Here's how the part is built. I have some questions about the finished solid (model axes, mm). Face numbers are marked on the shaded views. A direction names the side the tool comes from. Coordinates: 2 decimals unless noted, no trailing zeros. Write each loop counter-clockwise with the first axis right and the second up, starting at its lowest first coordinate (ties: lowest second). Pieces come first, ordered by that corner, then holes.
Item 1: I'm going to push flat-ended pins straight in: pin 1 Ø10 at (x, y) = (-18, 30) entering from -Z; pin 2 Ø4 at (y, z) = (29.5, 4) entering from -X; pin 3 Ø5.5 at (x, z) = (58.67, 4.78) entering from +Y; pin 4 Ø4.5 at (x, z) = (19.56, 4.95) entering from -Y. Where does each tip first touch, or does it pass through?
Item 2: If I drill on line 1 (X direction, y = 49, z = 5); line 2 (X direction, y = 45.5, z = 4.5); line 3 (Y direction, x = 19.5, z = 2), over which ranges is the centre line in solid material (lowest first)?
Item 3: If we section it at D-D (y = 31): Please give me the cut outline in (x, z), then the cut area to 3 significant figures.
Item 4: For the marked faces 1, 2 and 3, which set-ups out of +Z, -Z, +X, -X, +Y, -Y let a thin tool reach every point of the face, with its end or its side?
Item 5: If we section it at B-B (x = -55.5): Please give me the cut outline in (y, z), then the cut area to 3 significant figures.
Item 6: If we section it at A-A (y = 25): Please give me the cut outline in (x, z), then the cut area to 3 significant figures.
Item 7: If we section it at C-C (y = 50.5): Please give me the cut outline in (x, z), then the cut area to 3 significant figures.
from build123d import *
from build123d import SkipClean  # not in build123d's __all__

# Parameters (mm, degrees)
F1_DEPTH       = 10
F3_D           = 3.556
F3_CBORE_D     = 7.62
F3_CBORE_DEPTH = 13.75
F4_DEPTH       = 10.0010001
F6_D           = 3.556
F7_R           = 5


with BuildPart() as f1:
    # F0 (on Top) → F1 (new body)
    with BuildSketch(Plane.XY):
        with BuildLine():
            ThreePointArc((30, 32.8671568591), (40.2999174323, 18.8723780946), (44.4550334608, 2))
            Line((44.4550334608, 2), (44.4550334608, 7))
            Line((44.4550334608, 7), (49.002550954, 7))
            ThreePointArc((49.002550954, 7), (42.6890737127, 25.0577929106), (30, 39.3732142452))
            Line((30, 39.3732142452), (30, 32.8671568591))
        make_face()
        with BuildLine():
            ThreePointArc((20.7364413533, 39.3732142452), (25.5759421328, 36.4159468368), (30, 32.8671568591))
            Line((30, 32.8671568591), (30, 39.3732142452))
            Line((30, 39.3732142452), (20.7364413533, 39.3732142452))
        make_face()
        with BuildLine():
            ThreePointArc((-20.7364413533, 39.3732142452), (0, 44.5), (20.7364413533, 39.3732142452))
            Line((20.7364413533, 39.3732142452), (30, 39.3732142452))
            ThreePointArc((30, 39.3732142452), (15.8315491079, 46.9000218853), (-1.83e-08, 49.5))
            ThreePointArc((-1.83e-08, 49.5), (-15.8315491253, 46.9000218795), (-30, 39.3732142452))
            Line((-30, 39.3732142452), (-20.7364413533, 39.3732142452))
        make_face()
        with BuildLine():
            Line((-30, 39.3732142452), (-30, 32.8671568591))
            ThreePointArc((-30, 32.8671568591), (-25.5759421328, 36.4159468368), (-20.7364413533, 39.3732142452))
            Line((-20.7364413533, 39.3732142452), (-30, 39.3732142452))
        make_face()
        with BuildLine():
            ThreePointArc((-44.4550334608, 2), (-40.2999174323, 18.8723780946), (-30, 32.8671568591))
            Line((-30, 32.8671568591), (-30, 39.3732142452))
            ThreePointArc((-30, 39.3732142452), (-42.6890737127, 25.0577929106), (-49.002550954, 7))
            Line((-49.002550954, 7), (-44.4550334608, 7))
            Line((-44.4550334608, 7), (-44.4550334608, 2))
        make_face()
        with BuildLine():
            Line((-64.4550334608, 2), (-49.4595794564, 2))
            ThreePointArc((-49.4595794564, 2), (-49.2945005172, 4.5057983491), (-49.002550954, 7))
            Line((-49.002550954, 7), (-64.4550334608, 7))
            Line((-64.4550334608, 7), (-64.4550334608, 2))
        make_face()
        with BuildLine():
            Line((-49.4595794564, 2), (-44.4550334608, 2))
            Line((-44.4550334608, 2), (-44.4550334608, 7))
            Line((-44.4550334608, 7), (-49.002550954, 7))
            ThreePointArc((-49.002550954, 7), (-49.2945005172, 4.5057983491), (-49.4595794564, 2))
        make_face()
        with BuildLine():
            Line((44.4550334608, 7), (44.4550334608, 2))
            Line((44.4550334608, 2), (49.4595794564, 2))
            ThreePointArc((49.4595794564, 2), (49.2945005172, 4.5057983491), (49.002550954, 7))
            Line((49.002550954, 7), (44.4550334608, 7))
        make_face()
        with BuildLine():
            ThreePointArc((49.002550954, 7), (49.2945005172, 4.5057983491), (49.4595794564, 2))
            Line((49.4595794564, 2), (64.4550334608, 2))
            Line((64.4550334608, 2), (64.4550334608, 7))
            Line((64.4550334608, 7), (49.002550954, 7))
        make_face()
        with BuildLine():
            Line((-30, 49.5), (-30, 39.3732142452))
            ThreePointArc((-30, 39.3732142452), (-15.8315491253, 46.9000218795), (-1.83e-08, 49.5))
            Line((-1.83e-08, 49.5), (-30, 49.5))
        make_face()
        with BuildLine():
            ThreePointArc((-1.83e-08, 49.5), (15.8315491079, 46.9000218853), (30, 39.3732142452))
            Line((30, 39.3732142452), (30, 49.5))
            Line((30, 49.5), (-1.83e-08, 49.5))
        make_face()
        with BuildLine():
            Line((-30, 32.8671568591), (30, 32.8671568591))
            ThreePointArc((30, 32.8671568591), (25.5759421328, 36.4159468368), (20.7364413533, 39.3732142452))
            Line((20.7364413533, 39.3732142452), (-20.7364413533, 39.3732142452))
            ThreePointArc((-20.7364413533, 39.3732142452), (-25.5759421328, 36.4159468368), (-30, 32.8671568591))
        make_face()
        Polygon((-30, 49.5), (-1.83e-08, 49.5), (30, 49.5), (30, 54.5), (-30, 54.5), align=None)
    extrude(amount=F1_DEPTH)

    # F3 (through all)
    with Locations(Plane.XZ.offset(-32.8671568591)):
        with Locations((-19.558, 4.9517820589), (19.558, 4.9517820589)):
            CounterBoreHole(F3_D / 2, F3_CBORE_D / 2, F3_CBORE_DEPTH)

    # F0 (on Top) → F4 (cut, through all)
    with BuildSketch(Plane.XY):
        with BuildLine():
            Line((-30, 32.8671568591), (30, 32.8671568591))
            ThreePointArc((30, 32.8671568591), (25.5759421328, 36.4159468368), (20.7364413533, 39.3732142452))
            Line((20.7364413533, 39.3732142452), (-20.7364413533, 39.3732142452))
            ThreePointArc((-20.7364413533, 39.3732142452), (-25.5759421328, 36.4159468368), (-30, 32.8671568591))
        make_face()
    with SkipClean():  # cleaning this boolean's faces spoils the solid; the shape is the same uncleaned
        extrude(amount=F4_DEPTH, mode=Mode.SUBTRACT)

    # F6 (through all)
    with Locations(Plane.XZ.offset(-2)):
        with Locations((-58.674, 4.78035165), (58.674, 4.78035165)):
            Hole(F6_D / 2)

    # F7
    f7_edges = [f1.edges().sort_by_distance(p)[0] for p in [
        (-49.002551, 7, 5),
        (49.002551, 7, 5),
        (30, 39.373214, 5),
        (-30, 39.373214, 5),
    ]]
    fillet(f7_edges, radius=F7_R)


solid = f1.part
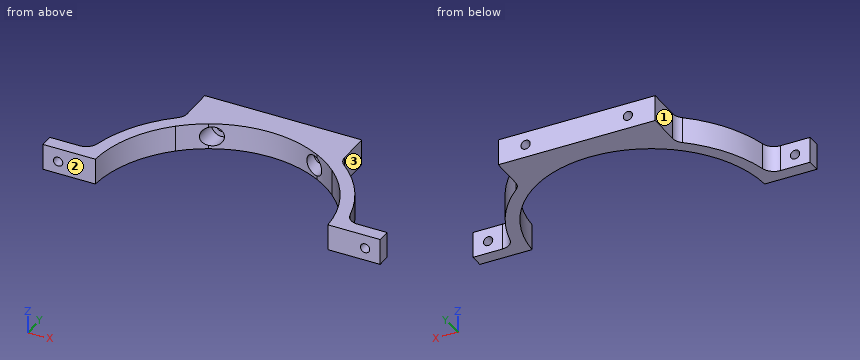
Answer list:
1. pin 1: passes through
1. pin 2: stops at x = -41.16
1. pin 3: stops at y = 7
1. pin 4: stops at y = 46.62
2. line 1: x = -30 to -21.34, -17.78 to 17.78, 21.34 to 30
2. line 2: x = -30 to -23.34, -15.77 to 15.77, 23.34 to 30
2. line 3: y = 46.62 to 54.5
3. outline: (-38.59, 0) - (-31.93, 0) - (-31.93, 10) - (-38.59, 10) - close; (31.93, 0) - (38.59, 0) - (38.59, 10) - (31.93, 10) - close
3. area: 133 mm2
4. face 1: +Z, -Z, -X, +Y
4. face 2: +Z, -Z, +X, -X, -Y
4. face 3: +Z, -Z, +X, +Y
5. outline: (2, 0) - (7, 0) - (7, 10) - (2, 10) - close
5. area: 50.0 mm2
6. outline: (-42.72, 0) - (-36.81, 0) - (-36.81, 10) - (-42.72, 10) - close; (36.81, 0) - (42.72, 0) - (42.72, 10) - (36.81, 10) - close
6. area: 118 mm2
7. outline: (-30, 0) - (30, 0) - (30, 10) - (-30, 10) - close; hole circle Ø3.56 at (-19.56, 4.95); hole circle Ø3.56 at (19.56, 4.95)
7. area: 580 mm2
